Geometry check sheet. Reference: the model listing, model coordinates, mm. A direction names the side the tool comes from. Give positions to 0.01 mm unless a question says otherwise; leave off trailing zeros. Loops run counter-clockwise (first coordinate to the right, second up) from the corner with the lowest first, then second, coordinate; pieces in that order, holes last. Notation, with made-up numbers: (-29, 43.5) -> (25, 43.5) arc R16 ccw to (25, 66.5) -> close; hole circle Ø7 at (6.5, -17.75). An arc over 180 degrees is marked (long way). Write item = value, one per line.
```python
from build123d import *

# Parameters (mm, degrees)
SKETCH005_W             = 58
SKETCH005_H             = 20
SKETCH005_R             = 2.75
PAD004_DEPTH            = 8
SKETCH006_R             = 2.25
PAD005_DEPTH            = 4
POCKET005_DEPTH         = 4
SKETCH011_W             = 15
SKETCH011_H             = 2.666667
POCKET007_DEPTH         = 20
SKETCH012_W             = 18
SKETCH012_H             = 3
POCKET008_DEPTH         = 8
FILLET_R                = 0.5
POCKET009_DEPTH         = 20
BODY002_PLACEMENT_ANGLE = 180


with BuildPart() as part:
    # Sketch005 → Pad004 (new body)
    with BuildSketch(Plane.XZ):
        Rectangle(SKETCH005_W, SKETCH005_H)
        Circle(SKETCH005_R, mode=Mode.SUBTRACT)
    extrude(amount=PAD004_DEPTH)

    # Sketch006 (on Face4 of Pad004) → Pad005 (join)
    with BuildSketch(Plane(origin=(-29, 0, 0), x_dir=(0, 0, -1), z_dir=(-1, 0, 0))):
        with BuildLine():
            Line((-10, 0), (10, 0))
            Line((10, 0), (10, 45.5))
            ThreePointArc((10, 45.5), (0, 55.5), (-10, 45.5))
            Line((-10, 45.5), (-10, 0))
        make_face()
        with Locations((0, 50)):
            Circle(SKETCH006_R, mode=Mode.SUBTRACT)
    pad005 = extrude(amount=PAD005_DEPTH)

    # Mirrored003: Pad005 across YZ
    add(pad005.mirror(Plane.YZ))

    # Sketch007 (on Face5 of Mirrored003) → Pocket005 (cut)
    with BuildSketch(Plane.XZ.offset(8)):
        Polygon((4.113621, 2.375), (0, 4.75), (-4.113621, 2.375), (-4.113621, -2.375), (0, -4.75), (4.113621, -2.375), align=None)
    extrude(amount=-POCKET005_DEPTH, mode=Mode.SUBTRACT)

    # Sketch011 (on Face14 of Pocket005) → Pocket007 (cut)
    with BuildSketch(Plane(origin=(0, 0, 10), x_dir=(-1, 0, 0), z_dir=(0, 0, 1))):
        with Locations((-19.5, 4.169504)):
            Rectangle(SKETCH011_W, SKETCH011_H)
    pocket007 = extrude(amount=-POCKET007_DEPTH, mode=Mode.SUBTRACT)

    # Mirrored004: Pocket007 across YZ
    add(pocket007.mirror(Plane.YZ), mode=Mode.SUBTRACT)

    # Sketch012 (on Face3 of Mirrored004) → Pocket008 (cut)
    with BuildSketch(Plane(origin=(0, 0, 0), x_dir=(1, 0, 0), z_dir=(0, 1, 0))):
        with Locations((0, 8.5)):
            Rectangle(SKETCH012_W, SKETCH012_H)
    extrude(amount=-POCKET008_DEPTH, mode=Mode.SUBTRACT)

    # Fillet
    fillet_edges = [part.edges().sort_by_distance(p)[0] for p in [
        (0, -8, -7),
        (9, -8, -8.5),
        (-9, -8, -8.5),
    ]]
    fillet(fillet_edges, radius=FILLET_R)

    # Sketch013 (on Face35 of Fillet) → Pocket009 (cut)
    with BuildSketch(Plane(origin=(0, 0, 10), x_dir=(-1, 0, 0), z_dir=(0, 0, 1))):
        Polygon((-29.221134, 0), (-32.431889, 2.958548), (-33, 4.069963), (-33, 0), align=None)
    extrude(amount=-POCKET009_DEPTH, mode=Mode.SUBTRACT)


with BuildPart() as part_1:
    # Body002 placement: moved
    add(part.part.moved(Location((0, -30, 9))).rotate(Axis((0, -30, 9), (1, 0, 0)), BODY002_PLACEMENT_ANGLE))


solid = part_1.part
```
Item 1: Section check A-A, the plane x = -24.5. Record the cut outline in (y, z).
Answer:
outline = (-30, -1) -> (-27.16, -1) -> (-27.16, 19) -> (-30, 19) -> close; (-24.5, -1) -> (-22, -1) -> (-22, 19) -> (-24.5, 19) -> close
Item 2: Section check C-C, the plane y = -6. Record the cut outline in (x, z).
Answer:
outline = (-33, -1) -> (-29, -1) -> (-29, 19) -> (-33, 19) -> close; (29, -1) -> (33, -1) -> (33, 19) -> (29, 19) -> close
Item 3: Thickness scan on L1, parallel to X at y = -25.5, z = 6.75; L2, parallel to X at y = 1, z = 0.75; L3, parallel to Y at x = -30.6, z = 9. Record the ranges inside material, lowest first. Write a range as [from, to].
Answer:
L1 = [-33, -27], [-12, -4.11], [4.11, 12], [27, 33]
L2 = [-33, -29], [29, 33]
L3 = [-30, 17.75], [22.25, 25.5]
Item 4: Tool access check on faces 1 (the flat face through (30, -14, 19)), 2 (the flat face through (9, -26, 17)), 3 (the flat face through (-2.03, -23.97, 5.42)), 4 (the flat face through (27, -26, 9)), 5 (the flat face through (-2.6, -22.3, -1)). Record the directions out of +Z, -Z, +X, -X, +Y, -Y that give a thin tool (end or side, any length) a straight path to the whole face; none if there is none.
Answer:
face_1 = +Z, +X, -X, +Y, -Y
face_2 = +Z, +Y, -Y
face_3 = +Y
face_4 = +Z, -Z
face_5 = -Z, +X, -X, +Y, -Y
Item 5: Gauge pin test, flat ends, axial feed: pin 1 (5 mm diameter, centred on x = -2, y = -21, fed in from +Z); pin 2 (3 mm diameter, centred on x = 6.5, z = 10.5, fed in from +Y); pin 3 (2.5 mm diameter, centred on x = -2, z = 8, fed in from +Y); pin 4 (2.5 mm diameter, centred on y = 20, z = 9, fed in from +X). Record the tip position at first contact, or that the pin passes through.
Answer:
pin_1 = 16
pin_2 = -22
pin_3 = -26
pin_4 = through
Item 6: Draft check along Z on faces 6 (the flat face through (0, -26, 16)), 7 (the flat face through (4.114, -24, 9)), 8 (the flat face through (-2.3, -30, 6.6)). Enter one of: +Z half, -Z half, draft (parallel to the pull), parting line (faces both ways), or undercut.
Answer:
face_6 = +Z half
face_7 = undercut
face_8 = draft
Item 7: Section check B-B, the plane z = 9. Give the number of separate pieces and of enclosed holes in the cut face, plus the area to 3 significant figures.
Answer:
separate_pieces = 4
enclosed_holes = 2
area = 730 mm^2
Item 8: Section check D-D, the plane y = 20. Record the cut outline in (x, z), plus the area to 3 significant figures.
Answer:
outline = (-33, 0.07) -> (-29, 0.07) -> (-29, 6.75) -> (-33, 6.75) -> close; (-33, 11.25) -> (-29, 11.25) -> (-29, 17.93) -> (-33, 17.93) -> close; (29, 0.07) -> (33, 0.07) -> (33, 6.75) -> (29, 6.75) -> close; (29, 11.25) -> (33, 11.25) -> (33, 17.93) -> (29, 17.93) -> close
area = 107 mm^2
